Print and shaded views of the part. All mm, measured from the part's lowest x, y and z. Round coordinates to 2 decimals unless told otherwise and drop trailing zeros. Write each loop counter-clockwise with the first axis right and the second up, starting at its lowest first coordinate (ties: lowest second). Pieces come first, ordered by that corner, then holes. Notation, with made-up numbers: M -22,81 L 35,81 A7 ccw 35,93 Z; hole C 77,-1.75 d9. An arc over 180 degrees is marked long. Write item = value, one per line.
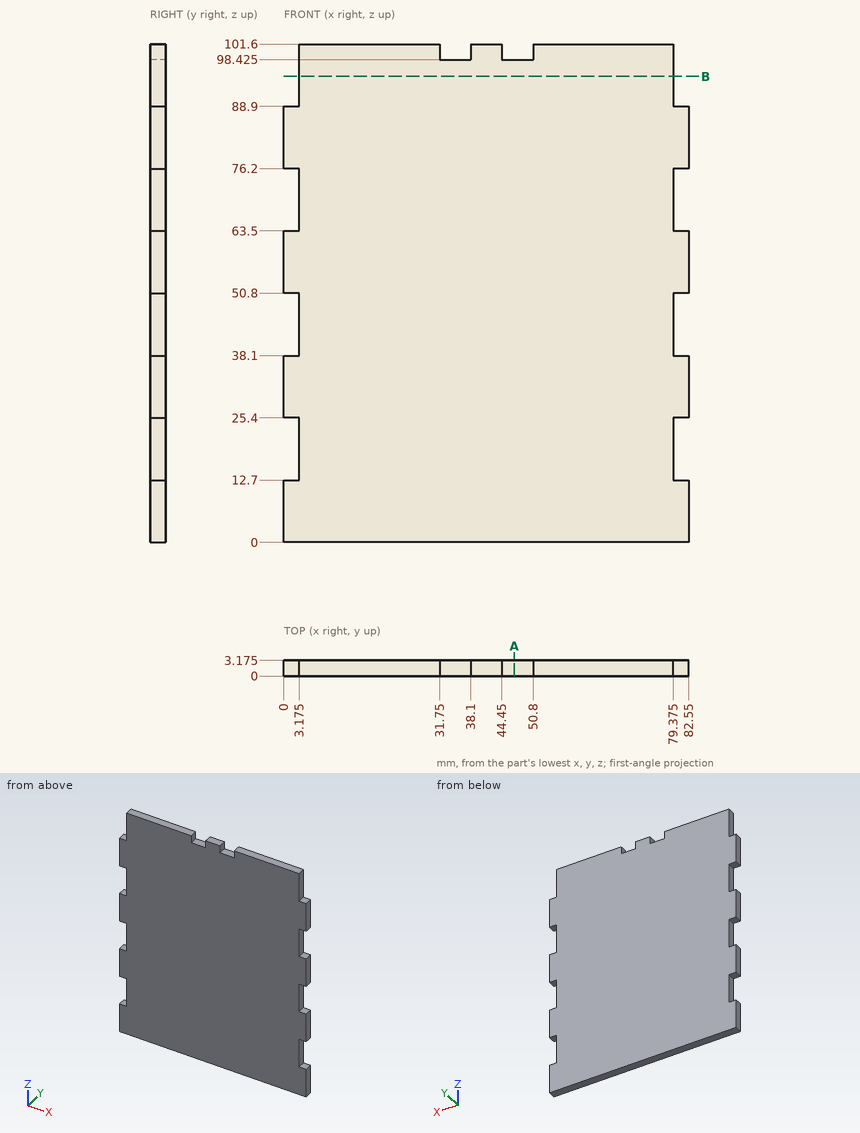
1. Probe probe 1 along X at (y, z) = (2.5, 38.5) (3 decimals); probe 2 along Z at (x, y) = (33, 1.05) (3 decimals). List the from-to ranges inside material, lowest first.
Responses:
probe_1 = 3.175 to 79.375
probe_2 = 0 to 98.425
2. Band-saw the part on A-A (x = 47). List the corners of the cut face in (y, z) (3 decimals), plus the area to 4 significant figures.
Responses:
outline = M 0,0 L 3.175,0 L 3.175,98.425 L 0,98.425 Z
area = 312.5 mm²
3. Flat gauge pins, fed straight in: pin 1 (1 mm diameter, centred on y = 1.5, z = 68, fed in from +X) (3 decimals); pin 2 (1 mm diameter, centred on x = 80, y = 1.5, fed in from +Z); pin 3 (1 mm diameter, centred on x = 49, y = 1, fed in from +Z) (3 decimals). Where does each tip first touch, or does it go through?
Responses:
pin_1 = 79.375
pin_2 = 88.9
pin_3 = 98.425
4. Band-saw the part on B-B (z = 95). List the corners of the cut face in (x, y) (3 decimals).
Responses:
outline = M 3.175,0 L 79.375,0 L 79.375,3.175 L 3.175,3.175 Z
